The model under review builds one solid part; all positions refer to its coordinate system, in mm. Give positions to 0.01 mm unless a question says otherwise; leave off trailing zeros. Write each loop counter-clockwise with the first axis right and the second up, starting at its lowest first coordinate (ties: lowest second). Pieces come first, ordered by that corner, then holes. Notation, with made-up numbers: (-26.75, 17.5) - (-6.75, 17.5) arc R26 cw to (-6.75, 42.5) - close; hole circle Ø9 at (52.25, 20). An arc over 180 degrees is marked (long way). One line per question, with ' | ' between items. Start each with the question number.
```python
from build123d import *

# Parameters (mm, degrees)
F0_R     = 3.175
F1_DEPTH = 20.6375
F2_SIZE  = 1.5875
F3_R     = 1.5875
F4_DEPTH = 12.7


with BuildPart() as f1:
    # F0 (on Top) → F1 (new body)
    with BuildSketch(Plane.XY):
        Circle(F0_R)
    extrude(amount=F1_DEPTH)

    # F2
    f2_edges = [f1.edges().sort_by_distance(p)[0] for p in [
        (-3.175, 0, 20.6375),
    ]]
    chamfer(f2_edges, length=F2_SIZE)

    # F3 (on Right) → F4 (cut, symmetric)
    with BuildSketch(Plane.YZ):
        with Locations((0, 10.31875)):
            Circle(F3_R)
    extrude(amount=F4_DEPTH, both=True, mode=Mode.SUBTRACT)


solid = f1.part
```
Item 1: The part is to be moulded in two halves that separate along Y. For faces 1 (the cylindrical face through (0.043, 1.514, 10.796)), 2 (the cylindrical face through (-2.52, -1.93, 9.39)), 3 (the flat face through (0, 0, 0)), say which applies: +Y half, -Y half, draft (parallel to the pull), parting line (faces both ways), or undercut.
Item 2: Clearance check with flat-ended pins moving along their axes: P1, Ø1.5, axis at x = 1, z = 17, coming from the -Y side; P2, Ø1.5, axis at y = -1, z = 12, coming from the +X side; P3, Ø1.9, axis at y = 0, z = 10.32, coming from the -X side. State where each tip first meets the part, or that it passes through.
Item 3: Take a section at C-C (z = 2). Give the boundary of the cut face in (x, y) (3 decimals), plus the area to 3 significant figures.
Item 4: For probe 1 along Z at (x, y) = (-1.5, 0); probe 2 along Z at (x, y) = (-2.25, 0.5); probe 3 along Y at (x, z) = (-1.75, 11.75), list the stretches that pass through material, from the lowest coordinate up.
Check sheet entries:
1) face 1: undercut | face 2: parting line | face 3: draft
2) P1: stops at y = -3.17 | P2: stops at x = 3.17 | P3: passes through
3) outline: circle Ø6.35 at (0, 0) | area: 31.7 mm^2
4) probe 1: z = 0 to 8.73, 11.91 to 20.64 | probe 2: z = 0 to 8.81, 11.83 to 19.92 | probe 3: y = -2.65 to -0.69, 0.69 to 2.65
